Source: CAD feature listing. Evaluate the final solid. Frame: model axes, mm. Face numbers are marked on the shaded views. Coordinates: 2 decimals unless noted, no trailing zeros. Loops run counter-clockwise (first coordinate to the right, second up) from the corner with the lowest first, then second, coordinate; pieces in that order, holes last. Notation, with made-up numbers: M -8,-24.75 L 7,-24.75 A20 ccw 7,0.25 Z; hole C 70,87 d2. An arc over 180 degrees is marked long. One line per question, with ' | ' between items. Start each with the question number.
1. Section query C-C, the plane y = -1. Output: boundary loops of the cut face in (x, z).
2. Mould query, pull axis X, two halves, no side actions, for the marked faces 1, 2, 3 and 4. Classes: pulls with the +X half, pulls with the -X half, needs draft (parallel to the pull), parting line crosses it, or undercut.
3. Ray query, probe 1 along Y at (x, z) = (8.25, -1.5) (3 decimals); probe 2 along Y at (x, z) = (11.25, 4.5) (3 decimals); probe 3 along Y at (x, z) = (-6.5, -3) (3 decimals). Return the intervals inside material, ascending.
4. Section query A-A, the plane z = 2.5. Output: boundary loops of the cut face in (x, y) (1 decimal).
5. Section query B-B, the plane y = 1. Output: boundary loops of the cut face in (x, z).
6. Section query D-D, the plane x = 9.75. Output: boundary loops of the cut face in (y, z) (3 decimals).
7. Pin query (flat end, axial travel): P1, Ø4, axis at y = -3, z = 2, coming from the +X side; P2, Ø1, axis at x = 7.5, y = 1, coming from the -Z side. Return the tip coordinate at first contact, or that it passes through.
```python
from build123d import *

# Parameters (mm, degrees)
SKETCH1_W                 = 25.4
SKETCH1_H                 = 18.542
BOSS_EXTRUDE1_DEPTH       = 4.445
TAP_DRILL_FOR_8_32_TAP1_D = 3.4544
FILLET1_R                 = 4.7625


with BuildPart() as part:
    # Sketch1 → Boss-Extrude1 (new, symmetric)
    with BuildSketch(Plane(origin=(0, 0, 0), x_dir=(1, 0, 0), z_dir=(0, 1, 0))):
        Rectangle(SKETCH1_W, SKETCH1_H)
    extrude(amount=BOSS_EXTRUDE1_DEPTH, both=True)

    # Tap Drill for #8-32 Tap1 (through all)
    with Locations(Plane.XY.offset(9.271)):
        with Locations((-6.985, 0), (6.985, 0)):
            Hole(TAP_DRILL_FOR_8_32_TAP1_D / 2)

    # Fillet1
    fillet1_edges = [part.edges().sort_by_distance(p)[0] for p in [
        (-12.7, -4.445, 0),
        (12.7, -4.445, 0),
    ]]
    fillet(fillet1_edges, radius=FILLET1_R)


solid = part.part
```
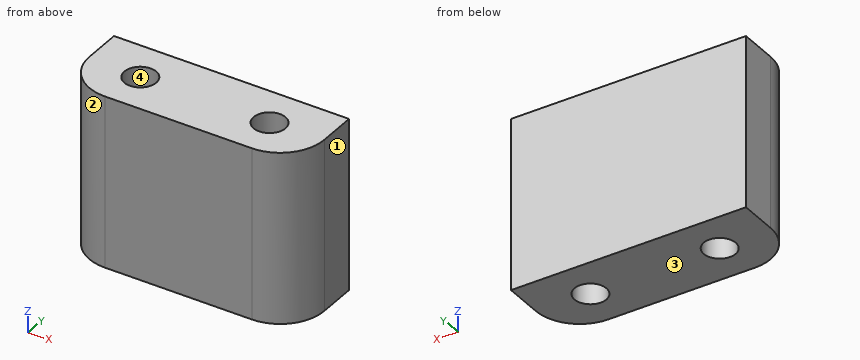
Taken from the geometry:
1) outline: M -12.51,-9.27 L -8.39,-9.27 L -8.39,9.27 L -12.51,9.27 Z; M -5.58,-9.27 L 5.58,-9.27 L 5.58,9.27 L -5.58,9.27 Z; M 8.39,-9.27 L 12.51,-9.27 L 12.51,9.27 L 8.39,9.27 Z
2) face 1: pulls with the +X half | face 2: pulls with the -X half | face 3: needs draft | face 4: undercut
3) probe 1: -4.435 to -1.176, 1.176 to 4.445 | probe 2: -3.104 to 4.445 | probe 3: -4.445 to -1.658, 1.658 to 4.445
4) outline: M -12.7,0.3 A4.8 ccw -7.9,-4.4 L 7.9,-4.4 A4.8 ccw 12.7,0.3 L 12.7,4.4 L -12.7,4.4 Z; hole C -7,0 d3.5; hole C 7,0 d3.5
5) outline: M -12.7,-9.27 L -8.39,-9.27 L -8.39,9.27 L -12.7,9.27 Z; M -5.58,-9.27 L 5.58,-9.27 L 5.58,9.27 L -5.58,9.27 Z; M 8.39,-9.27 L 12.7,-9.27 L 12.7,9.27 L 8.39,9.27 Z
6) outline: M -4.087,-9.271 L 4.445,-9.271 L 4.445,9.271 L -4.087,9.271 Z
7) P1: x = 12.51 | P2: through
